```python
from build123d import *

# Parameters (mm, degrees)
SKETCH_1_W          = 140.7
SKETCH_1_H          = 78.95
SKETCH_1_R          = 1.7
EXTRUDE_1_DEPTH     = 7
SKETCH_2_W          = 120.7
SKETCH_2_H          = 58.95
CUT_EXTRUDE_1_DEPTH = 5


with BuildPart() as part:
    # 草图1 → 凸台-拉伸1 (new body)
    with BuildSketch(Plane.XY):
        Rectangle(SKETCH_1_W, SKETCH_1_H)
        with Locations((-66.25272379, 35.66826865)):
            Circle(SKETCH_1_R, mode=Mode.SUBTRACT)
        with Locations(Location((66.25272379, 35.66826865, 0), (0, 0, 180))):
            Circle(SKETCH_1_R, mode=Mode.SUBTRACT)
        with Locations((66.25272379, -35.66826865)):
            Circle(SKETCH_1_R, mode=Mode.SUBTRACT)
        with Locations(Location((-66.25272379, -35.66826865, 0), (0, 0, 180))):
            Circle(SKETCH_1_R, mode=Mode.SUBTRACT)
    extrude(amount=EXTRUDE_1_DEPTH)

    # 草图2 → 切除-拉伸1 (cut)
    with BuildSketch(Plane.XY.offset(7)):
        Rectangle(SKETCH_2_W, SKETCH_2_H)
    extrude(amount=-CUT_EXTRUDE_1_DEPTH, mode=Mode.SUBTRACT)


solid = part.part
```
Here's how the part is built. I have some questions about the finished solid (model axes, mm). A direction names the side the tool comes from. Give positions to 0.01 mm unless a question says otherwise; leave off trailing zeros. Order: outer loops, then holes, each group sorted by start corner. A loop starts at its lowest first (then second) coordinate and runs counter-clockwise, first axis right, second up. Notation, with made-up numbers: M 79,32.25 L 112,32.25 A20 ccw 112,45.25 Z; hole C 71,42 d4. An arc over 180 degrees is marked long. Use a Markdown table: item, result. Add a question column.
1. Suppose I cut it at A-A (x = -59). List the corners of the cut face in (y, z) for me (3 decimals), and give its area (3 significant figures).
2. If we mould it in two halves opening along X, with no side actions, what happens to faces 3 (the flat face through (-1, 39.475, 3)), 4 (the cylindrical face through (65.339, 34.235, 3.451)), 5 (the flat face through (70.35, -1, 3))? For each: +X half, -X half, draft (parallel to the pull), parting line (faces both ways), or undercut.
3. For pin 1 Ø4.5 at (x, y) = (66.25, 35.67) entering from -Z; pin 2 Ø1.5 at (x, y) = (17.5, 1) entering from +Z, each with a flat end and sliding along its axis, tell me the tip position at first contact or that it passes through.
4. Suppose I cut it at B-B (y = -15). List the corners of the cut face in (x, z) for me, and give its area (3 significant figures).
5. On a 3-axis mill with a long thin cutter (end or side, diameter ignored), from which of +Z, -Z, +X, -X, +Y, -Y can I reach the whole of each face in a straight line? I mean faces 1 (the flat face through (-1, -39.475, 3)), 2 (the flat face through (-60.35, 0, 5)). Say none if no direction works.
6. Suppose I cut it at C-C (z = 3.5). List the corners of the cut face in (x, y) for me (3 decimals).
7. I need wall thicknesses on probe 1 along X at (y, z) = (36, 6); probe 2 along Y at (x, z) = (12, 5.5) (3 decimals); probe 3 along X at (y, z) = (-19, 3.25). Which ranges of each line are inside material? Lowest first, please. Write a range as from..to.
Results list:
| question | item | result |
|---|---|---|
| 1 | outline | M -39.475,0 L 39.475,0 L 39.475,7 L 29.475,7 L 29.475,2 L -29.475,2 L -29.475,7 L -39.475,7 Z |
| 1 | area | 258 mm² |
| 2 | face 3 | draft |
| 2 | face 4 | undercut |
| 2 | face 5 | +X half |
| 3 | pin 1 | stops at z = 0 |
| 3 | pin 2 | stops at z = 2 |
| 4 | outline | M -70.35,0 L 70.35,0 L 70.35,7 L 60.35,7 L 60.35,2 L -60.35,2 L -60.35,7 L -70.35,7 Z |
| 4 | area | 381 mm² |
| 5 | face 1 | +Z, -Z, +X, -X, -Y |
| 5 | face 2 | +Z |
| 6 | outline | M -70.35,-39.475 L 70.35,-39.475 L 70.35,39.475 L -70.35,39.475 Z; hole C -66.253,-35.668 d3.4; hole C -66.253,35.668 d3.4; hole M -60.35,-29.475 L 60.35,-29.475 L 60.35,29.475 L -60.35,29.475 Z; hole C 66.253,-35.668 d3.4; hole C 66.253,35.668 d3.4 |
| 7 | probe 1 | x = -70.35..-67.92, -64.59..64.59, 67.92..70.35 |
| 7 | probe 2 | y = -39.475..-29.475, 29.475..39.475 |
| 7 | probe 3 | x = -70.35..-60.35, 60.35..70.35 |
